Design review of the part built by this model. Coordinates are the model's own, in mm. A direction names the side the tool comes from. Round coordinates to 2 decimals unless told otherwise and drop trailing zeros. Loops run counter-clockwise (first coordinate to the right, second up) from the corner with the lowest first, then second, coordinate; pieces in that order, holes last. Notation, with made-up numbers: (-33.5, 0.25) - (5.5, 0.25) arc R27 ccw to (5.5, 21.25) - close; hole circle Ø3 at (4, 42). An arc over 180 degrees is marked (long way). Return JSON: item names as keys, results as strings. Group by question number.
(1) The part is to be moulded in two halves that separate along Z. For faces 6 (the flat face through (0, 253, -1850)), 7 (the cylindrical face through (420.3, 537.8, 151.5)), 8 (the flat face through (440, 560, 140)), say which applies: pulls with the +Z half, pulls with the -Z half, needs draft (parallel to the pull), parting line crosses it, or undercut.
(2) Clearance check with flat-ended pins moving along their axes: pin 1 (1 mm diameter, centred on x = 36, y = 254.5, fed in from -Z); pin 2 (10 mm diameter, centred on x = 406, z = 100.5, fed in from +Y); pin 3 (11 mm diameter, centred on y = 556, z = 90, fed in from +X). State where each tip first meets the part, or that it passes through.
(3) We need section B-B, the plane z = 140. Write out the cut boundary in (x, y), and give its area (3 significant figures).
(4) We need section A-A, the plane y = 256.5. Write out the cut boundary in (x, z), and give its area (3 significant figures).
(5) For faces 1 (the flat face through (400, -114, 45)), 2 (the flat face through (440, -140, 140)), 3 (the flat face through (-2, 40, -604)), 4 (the flat face through (40, 0, -912)), 5 (the flat face through (400, 329, 45)), list the 3-axis set-ups (+Z, -Z, +X, -X, +Y, -Y) from which the entire face can be reached by the end or side of a thin tool; tool diameter is ignored.
(6) We need section C-C, the plane z = -1583.5. Write out the cut boundary in (x, y), and give its area (3 significant figures).
(7) We need section D-D, the plane x = -285.5. Write out the cut boundary in (y, z), and give its area (3 significant figures).
(8) Wall thickness on L1, parallel to Y at x = -20, z = 48; L2, parallel to Z at x = 86, y = -0.5: over which ranges is each line inside the solid? List them lowest first. Write a range as [from, to].
from build123d import *

# Parameters (mm, degrees)
SKETCH_1_W          = 800
SKETCH_1_H          = 80
EXTRUDE_1_DEPTH     = 80
SKETCH_2_W          = 80
SKETCH_2_H          = 80
EXTRUDE_2_DEPTH     = 1850
SKETCH_3_W          = 80
SKETCH_3_H          = 500
EXTRUDE_3_DEPTH     = 40
SKETCH_4_W          = 80
SKETCH_4_H          = 800
EXTRUDE_4_DEPTH     = 40
SKETCH_5_R          = 4
CUT_EXTRUDE_1_DEPTH = 40
SKETCH_7_R          = 4
CUT_EXTRUDE_2_DEPTH = 40
FILLET_1_R          = 10
FILLET_2_R          = 10
SKETCH_9_R          = 25
EXTRUDE_5_DEPTH     = 40
EXTRUDE_5_2_DEPTH   = 40
SKETCH_10_W         = 60
SKETCH_10_H         = 10
EXTRUDE_1_2_DEPTH   = 20


with BuildPart() as part:
    # 草图1 → Extrude 1 (new body)
    with BuildSketch(Plane.XY):
        Rectangle(SKETCH_1_W, SKETCH_1_H)
    extrude(amount=EXTRUDE_1_DEPTH)

    # 草图7 → 切除-拉伸2 (cut)
    with BuildSketch(Plane.XY.offset(80)):
        with Locations((-20, 20)):
            Circle(SKETCH_7_R)
        with Locations((20, 20)):
            Circle(SKETCH_7_R)
    extrude(amount=-CUT_EXTRUDE_2_DEPTH, mode=Mode.SUBTRACT)


with BuildPart() as body_2:
    # 草图2 → 凸台-拉伸2 (new body)
    with BuildSketch(Plane(origin=(0, 0, 0), x_dir=(-1, 0, 0), z_dir=(0, 0, -1))):
        Rectangle(SKETCH_2_W, SKETCH_2_H)
    extrude(amount=EXTRUDE_2_DEPTH)

    # 圆角1
    fillet_1_edges = [body_2.edges().sort_by_distance(p)[0] for p in [
        (40, 40, -925),
        (-40, 40, -925),
        (-40, -40, -925),
        (40, -40, -925),
    ]]
    fillet(fillet_1_edges, radius=FILLET_1_R)


with BuildPart() as body_3:
    # 草图3 → 凸台-拉伸3 (new body)
    with BuildSketch(Plane(origin=(0, 0, -1850), x_dir=(-1, 0, 0), z_dir=(0, 0, -1))):
        with Locations((0, 210)):
            Rectangle(SKETCH_3_W, SKETCH_3_H)
    extrude(amount=EXTRUDE_3_DEPTH)

    # 圆角2
    fillet_2_edges = [body_3.edges().sort_by_distance(p)[0] for p in [
        (-40, 210, -1890),
        (40, 210, -1890),
        (-40, 210, -1850),
        (40, 210, -1850),
    ]]
    fillet(fillet_2_edges, radius=FILLET_2_R)


with BuildPart() as body_4:
    # 草图4 → 凸台-拉伸4 (new body)
    with BuildSketch(Plane.ZY.offset(400)):
        with Locations((40, 210)):
            Rectangle(SKETCH_4_W, SKETCH_4_H)
    extrude(amount=EXTRUDE_4_DEPTH)


with BuildPart() as body_5:
    # 镜向2: mirrored copy
    add(body_4.part.mirror(Plane(origin=(0, 0, 0), x_dir=(0, 0, 1), z_dir=(1, 0, 0))))

    # 草图5 → 切除-拉伸1 (cut)
    with BuildSketch(Plane(origin=(440, 0, 0), x_dir=(0, 0, -1), z_dir=(1, 0, 0))):
        with Locations((-20, 20)):
            Circle(SKETCH_5_R)
        with Locations((-20, -20)):
            Circle(SKETCH_5_R)
    extrude(amount=-CUT_EXTRUDE_1_DEPTH, mode=Mode.SUBTRACT)


with BuildPart() as body_6:
    # 草图9 → 凸台-拉伸5 (new body)
    with BuildSketch(Plane.ZY.offset(440)):
        with Locations((140, 560)):
            Circle(SKETCH_9_R)
    extrude(amount=-EXTRUDE_5_DEPTH)


with BuildPart() as body_7:
    # 草图9 → Extrude 5 2 (new body)
    with BuildSketch(Plane.ZY.offset(440)):
        with Locations((140, -140)):
            Circle(SKETCH_9_R)
    extrude(amount=-EXTRUDE_5_2_DEPTH)


with BuildPart() as body_4_1:
    add(body_4.part)

    add(body_6.part)  # Extrude 1 2 merges body 6

    add(body_7.part)  # Extrude 1 2 merges body 7
    # 草图10 → Extrude 1 2 (add)
    with BuildSketch(Plane(origin=(-400, 0, 0), x_dir=(0, 0, -1), z_dir=(1, 0, 0))):
        with Locations((-110, 555)):
            Rectangle(SKETCH_10_W, SKETCH_10_H)
        with Locations((-110, -145)):
            Rectangle(SKETCH_10_W, SKETCH_10_H)
    extrude(amount=-EXTRUDE_1_2_DEPTH)


with BuildPart() as body_6_2:
    # 镜向6: mirrored copy
    add(body_4_1.part.mirror(Plane(origin=(0, 0, 0), x_dir=(0, 0, 1), z_dir=(1, 0, 0))))


with BuildPart() as part_1:
    add(part.part)

    # Combine 1: union body 5, body 6 2, body 2, body 4
    add(body_5.part)
    add(body_6_2.part)
    add(body_2.part)
    add(body_4_1.part)

    # Combine 2: union body 3
    add(body_3.part)


solid = part_1.part
Solutions:
{
 "1": {"face 6": "pulls with the +Z half", "face 7": "undercut", "face 8": "needs draft"},
 "2": {"pin 1": "z = -1888.35", "pin 2": "y = 560", "pin 3": "x = 420"},
 "3": {"outline": "(-440, -165) - (-400, -165) - (-400, -115) - (-440, -115) - close; (-440, 535) - (-400, 535) - (-400, 585) - (-440, 585) - close; (400, -165) - (440, -165) - (440, -115) - (400, -115) - close; (400, 535) - (440, 535) - (440, 585) - (400, 585) - close", "area": "8,000 mm^2"},
 "4": {"outline": "(-440, 0) - (-400, 0) - (-400, 80) - (-440, 80) - close; (-40, -1880) arc R10 ccw to (-30, -1890) - (30, -1890) arc R10 ccw to (40, -1880) - (40, -1860) arc R10 ccw to (30, -1850) - (-30, -1850) arc R10 ccw to (-40, -1860) - close; (400, 0) - (440, 0) - (440, 80) - (400, 80) - close", "area": "9,510 mm^2"},
 "5": {"face 1": "+Z, -Z, -Y", "face 2": "+Z, -Z, +X, +Y, -Y", "face 3": "+Z, +Y", "face 4": "-Z, +X, +Y, -Y", "face 5": "+Z, -Z, +Y"},
 "6": {"outline": "(-40, -30) arc R10 ccw to (-30, -40) - (30, -40) arc R10 ccw to (40, -30) - (40, 30) arc R10 ccw to (30, 40) - (-30, 40) arc R10 ccw to (-40, 30) - close", "area": "6,310 mm^2"},
 "7": {"outline": "(-40, 0) - (40, 0) - (40, 80) - (-40, 80) - close", "area": "6,400 mm^2"},
 "8": {"L1": "[-40, 16], [24, 40]", "L2": "[0, 80]"}
}
